```python
from build123d import *

# Parameters (mm, degrees)
SKETCH_1_R                = 44
EXTRUDE_1_DEPTH           = 80
CUT_EXTRUDE_START         = 5
SKETCH_2_W                = 23
SKETCH_2_H                = 72
CUT_EXTRUDE_5_DEPTH       = 97.350875675
SKETCH_3_W                = 20.9
SKETCH_3_H                = 40.9
CUT_EXTRUDE_6_DEPTH       = 120.436175424
EXTRUDE_2_DEPTH           = 75
SKETCH_7_R                = 6.5
CUT_EXTRUDE_7_DEPTH       = 4
CUT_EXTRUDE_START_2       = -4
SKETCH_8_R                = 6.5
CUT_EXTRUDE_8_DEPTH       = 4
CUT_EXTRUDE_9_REACH       = 105.057
SKETCH_9_R                = 5.5
CUT_EXTRUDE_10_DEPTH      = 120.436175424
CUT_EXTRUDE_10_DEPTH_BACK = 120.436175424
CUT_EXTRUDE_START_3       = -12
CUT_EXTRUDE_13_DEPTH      = 12
CUT_EXTRUDE_14_REACH      = 96.265
CUT_REVOLVE_1_ANGLE       = 180
CUT_REVOLVE_2_ANGLE       = 180
CUT_EXTRUDE_20_REACH      = 93.901


with BuildPart() as part:
    # 草图1 → 凸台-拉伸1 (new body)
    with BuildSketch(Plane(origin=(0, 0, 0), x_dir=(1, 0, 0), z_dir=(0, 1, 0))):
        with Locations(Location((0, 0, 0), (0, 0, 270))):
            Circle(SKETCH_1_R)
    extrude(amount=EXTRUDE_1_DEPTH)

    # 草图2 → 切除-拉伸5 (cut, through all)
    with BuildSketch(Plane(origin=(0, 0, 0), x_dir=(1, 0, 0), z_dir=(0, 1, 0)).offset(CUT_EXTRUDE_START)):
        with BuildLine():
            Line((33, 29.103264422), (33, -19.45))
            Line((33, -19.45), (39.467676648, -19.45))
            ThreePointArc((39.467676648, -19.45), (43.614744195, 5.809826917), (33, 29.103264422))
        make_face()
        with Locations((11.5, 8)):
            Rectangle(SKETCH_2_W, SKETCH_2_H)
    cut_extrude_5 = extrude(amount=CUT_EXTRUDE_5_DEPTH, mode=Mode.SUBTRACT)

    # 镜向1: 切除-拉伸5 across plane
    add(cut_extrude_5.mirror(Plane(origin=(0, 0, 0), x_dir=(0, 0, 1), z_dir=(1, 0, 0))), mode=Mode.SUBTRACT)

    # 草图3 → 切除-拉伸6 (cut, through all)
    with BuildSketch(Plane(origin=(33, 0, 0), x_dir=(0, 0, -1), z_dir=(1, 0, 0))):
        with Locations((-7, 33)):
            Rectangle(SKETCH_3_W, SKETCH_3_H)
    extrude(amount=-CUT_EXTRUDE_6_DEPTH, mode=Mode.SUBTRACT)

    # 草图6 → 凸台-拉伸2 (add)
    with BuildSketch(Plane(origin=(0, 5, 0), x_dir=(1, 0, 0), z_dir=(0, 1, 0))):
        with BuildLine():
            Line((-8.2, 43.229156827), (-8.2, -28))
            Line((-8.2, -28), (3.8, -28))
            Line((3.8, -28), (3.8, 43.835601969))
            ThreePointArc((3.8, 43.835601969), (-2.220798038, 43.943919444), (-8.2, 43.229156827))
        make_face()
    extrude(amount=EXTRUDE_2_DEPTH)

    # 草图7 → 切除-拉伸7 (cut)
    with BuildSketch(Plane(origin=(3.8, 0, 0), x_dir=(0, 0, -1), z_dir=(1, 0, 0))):
        with Locations((-7, 43)):
            Circle(SKETCH_7_R)
    extrude(amount=-CUT_EXTRUDE_7_DEPTH, mode=Mode.SUBTRACT)

    # 草图8 → 切除-拉伸8 (cut)
    with BuildSketch(Plane.ZY.offset(8.2).offset(CUT_EXTRUDE_START_2)):
        with Locations(Location((7, 43, 0), (0, 0, 180))):
            Circle(SKETCH_8_R)
    extrude(amount=CUT_EXTRUDE_8_DEPTH, mode=Mode.SUBTRACT)

    # 草图9 → 切除-拉伸9 (cut, up to next)
    with BuildSketch(Plane(origin=(3.8, 0, 0), x_dir=(0, 0, -1), z_dir=(1, 0, 0)), mode=Mode.PRIVATE) as cut_extrude_9_sk1:
        with Locations((-7, 43)):
            Circle(SKETCH_9_R)
    cut_extrude_9_tool1 = extrude(cut_extrude_9_sk1.sketch, amount=-CUT_EXTRUDE_9_REACH, mode=Mode.PRIVATE) & part.part
    add(cut_extrude_9_tool1.solids().sort_by_distance((3.8, 43, 7))[0], mode=Mode.SUBTRACT)

    # 草图10 → 切除-拉伸10 (cut, two sides: drawn at the far end of the back side and taken through both)
    with BuildSketch(Plane(origin=(33, 0, 0), x_dir=(0, 0, -1), z_dir=(1, 0, 0)).offset(-CUT_EXTRUDE_10_DEPTH_BACK)):
        with BuildLine():
            Line((44, 80), (44, 65))
            Line((44, 65), (-7, 65))
            ThreePointArc((-7, 65), (-19.069252989, 61.393834083), (-27.181803363, 51.757557481))
            Line((-27.181803363, 51.757557481), (-44, 13))
            Line((-44, 13), (-44, 80))
            Line((-44, 80), (44, 80))
        make_face()
    extrude(amount=CUT_EXTRUDE_10_DEPTH + CUT_EXTRUDE_10_DEPTH_BACK, mode=Mode.SUBTRACT)

    # 草图18 → 切除-拉伸13 (cut)
    with BuildSketch(Plane.ZY.offset(8.2).offset(CUT_EXTRUDE_START_3)):
        with BuildLine():
            ThreePointArc((-16.994306564, 43.522735592), (-16.113193955, 49.463765557), (-13.784609691, 55))
            ThreePointArc((-13.784609691, 55), (-8.989980812, 60.897500207), (-2.591663047, 65))
            Line((-2.591663047, 65), (-21.495613698, 65))
            ThreePointArc((-21.495613698, 65), (-26.943692062, 54.992738185), (-28.991459846, 43.784103388))
            Line((-28.991459846, 43.784103388), (-16.994306564, 43.522735592))
        make_face()
    extrude(amount=CUT_EXTRUDE_13_DEPTH, mode=Mode.SUBTRACT)

    # 草图19 → 切除-拉伸14 (cut, up to next)
    with BuildSketch(Plane.ZY.offset(8.2), mode=Mode.PRIVATE) as cut_extrude_14_sk1:
        with BuildLine():
            Line((-25.784609691, 34.215390309), (-20.368569743, 43.596246675))
            Line((-20.368569743, 43.596246675), (-28.991459846, 43.784103388))
            ThreePointArc((-28.991459846, 43.784103388), (-26.943692062, 54.992738185), (-21.495613698, 65))
            Line((-21.495613698, 65), (-43.229156827, 65))
            Line((-43.229156827, 65), (-43.229156827, 44.287004294))
            Line((-43.229156827, 44.287004294), (-25.784609691, 34.215390309))
        make_face()
    cut_extrude_14_tool1 = extrude(cut_extrude_14_sk1.sketch, amount=-CUT_EXTRUDE_14_REACH, mode=Mode.PRIVATE) & part.part
    # 草图19 → 切除-拉伸14 (cut, up to next)
    with BuildSketch(Plane.ZY.offset(8.2), mode=Mode.PRIVATE) as cut_extrude_14_sk2:
        with BuildLine():
            Line((-20.368569743, 43.596246675), (-13.784609691, 55))
            Line((-13.784609691, 55), (-13.784609691, 93.841822502))
            Line((-13.784609691, 93.841822502), (-75.156898342, 93.841822502))
            Line((-75.156898342, 93.841822502), (-75.156898342, 62.720494453))
            Line((-75.156898342, 62.720494453), (-43.229156827, 44.287004294))
            Line((-43.229156827, 44.287004294), (-43.229156827, 65))
            Line((-43.229156827, 65), (-21.495613698, 65))
            ThreePointArc((-21.495613698, 65), (-26.943692062, 54.992738185), (-28.991459846, 43.784103388))
            Line((-28.991459846, 43.784103388), (-20.368569743, 43.596246675))
        make_face()
    cut_extrude_14_tool2 = extrude(cut_extrude_14_sk2.sketch, amount=-CUT_EXTRUDE_14_REACH, mode=Mode.PRIVATE) & part.part
    add(cut_extrude_14_tool1.solids().sort_by_distance((-8.2, 51.836761, -33.537679))[0], mode=Mode.SUBTRACT)
    add(cut_extrude_14_tool2.solids().sort_by_distance((-8.2, 73.617285, -43.768646))[0], mode=Mode.SUBTRACT)

    # 草图24 → 切除-旋转1 (revolve, symmetric, cut)
    with BuildSketch(Plane(origin=(0, 43, 0), x_dir=(-1, 0, 0), z_dir=(0, -1, 0))) as cut_revolve_1_sk:
        Polygon((15.5, -31.8), (15.5, -34.8), (-15.5, -34.8), (-15.5, -31.8), (-15.5, -7), (-3.8, -7), (-3.8, -31.8), (8.2, -31.8), (8.2, -7), (15.5, -7), align=None)
    revolve(axis=Axis((-101.499852898, 43, 7), (1, 0, 0)), revolution_arc=CUT_REVOLVE_1_ANGLE / 2, mode=Mode.SUBTRACT)
    revolve(cut_revolve_1_sk.sketch, axis=Axis((-101.499852898, 43, 7), (-1, 0, 0)), revolution_arc=CUT_REVOLVE_1_ANGLE / 2, mode=Mode.SUBTRACT)

    # 草图26 → 切除-旋转2 (revolve, symmetric, cut)
    with BuildSketch(Plane(origin=(0, 43, 0), x_dir=(1, 0, 0), z_dir=(0, 1, 0))) as cut_revolve_2_sk:
        Polygon((-15.5, -34.551556537), (-23, -29.3), (-23, -28), (-15.5, -28), align=None)
        Polygon((15.5, -34.551556537), (23, -29.3), (23, -28), (15.5, -28), align=None)
    revolve(axis=Axis((-28, 43, 7), (1, 0, 0)), revolution_arc=CUT_REVOLVE_2_ANGLE / 2, mode=Mode.SUBTRACT)
    revolve(cut_revolve_2_sk.sketch, axis=Axis((-28, 43, 7), (-1, 0, 0)), revolution_arc=CUT_REVOLVE_2_ANGLE / 2, mode=Mode.SUBTRACT)

    # 草图28 → 切除-拉伸20 (cut, up to next)
    with BuildSketch(Plane(origin=(3.8, 0, 0), x_dir=(0, 0, -1), z_dir=(1, 0, 0)), mode=Mode.PRIVATE) as cut_extrude_20_sk1:
        with BuildLine():
            ThreePointArc((-7, 15.2), (-6.737382717, 15.201240456), (-6.474788871, 15.204961715))
            Line((-6.474788871, 15.204961715), (-5.365047446, 18.253951222))
            ThreePointArc((-5.365047446, 18.253951222), (-6.182078765, 18.213491475), (-7, 18.2))
            Line((-7, 18.2), (-7, 15.2))
        make_face()
    cut_extrude_20_tool1 = extrude(cut_extrude_20_sk1.sketch, amount=-CUT_EXTRUDE_20_REACH, mode=Mode.PRIVATE) & part.part
    add(cut_extrude_20_tool1.solids().sort_by_distance((3.8, 16.966985, 6.413126))[0], mode=Mode.SUBTRACT)


solid = part.part
```
Check sheet for the modelled part. Datum: model origin and axes. Units: mm. A direction names the side the tool comes from. Coordinates: 2 decimals unless noted, no trailing zeros. Order: outer loops, then holes, each group sorted by start corner. A loop starts at its lowest first (then second) coordinate and runs counter-clockwise, first axis right, second up. Notation, with made-up numbers: (45.25, -35.75) -> (77.25, -35.75) arc R30 cw to (77.25, -6.75) -> close; hole circle Ø8 at (16, 29). An arc over 180 degrees is marked (long way). Write each question's results on one line, items separated by ' | '. Start each with the question number.
1) Section check B-B (x = -27.5). Enter the section's corners in (y, z).
2) Section check D-D (z = -32.5). Enter the section's corners in (x, y).
3) Section check A-A (y = 21). Enter the section's corners in (x, z).
4) Draft check along Z on faces 1 (the face through (-2.28, 46.58, 29.43)), 2 (the face through (-2.284, 38.84, -23.115)), 3 (the face through (23, 35, -4)). Enter one of: pulls with the +Z half, pulls with the -Z half, needs draft (parallel to the pull), parting line crosses it, or undercut.
5) Depth check by flat-ended pin: pin 1 (10 mm diameter, centred on x = -26, y = 10, fed in from -Z); pin 2 (15.5 mm diameter, centred on x = 11, y = 18.5, fed in from -Z); pin 3 (4 mm diameter, centred on y = 43.5, z = -22.5, fed in from -X). Enter the tip coordinate at first touch or a pass-through.
6) Material ranges on line 1 along X through (y, z) = (10.5, -4); line 2 along X through (y, z) = (7.5, 19.5); line 3 along Z through (x, y) = (-6.8, 43), recorded low to high.
7) Set-up check for faces 4 (the face through (37, 5, -5)), 5 (the face through (-15, 5, -8)), 6 (the face through (-28, 53.45, 7)): record each of +Z, -Z, +X, -X, +Y, -Y from which the full face is reachable in a straight line by a thin tool's end or side.
8) Section check C-C (z = 22.5). Enter the section's corners in (x, y), and give its area (3 significant figures).
Checked values:
1) outline: (0, -34.35) -> (65, -34.35) -> (65, 7) arc R22 ccw to (51.76, 27.18) -> (35.24, 34.35) -> (0, 34.35) -> close; hole (12.55, -3.45) -> (53.45, -3.45) -> (53.45, 17.45) -> (12.55, 17.45) -> close
2) outline: (-29.66, 0) -> (29.66, 0) -> (29.66, 65) -> (23, 65) -> (23, 5) -> (3.8, 5) -> (3.8, 38.09) -> (-8.2, 38.09) -> (-8.2, 5) -> (-23, 5) -> (-23, 65) -> (-29.66, 65) -> close
3) outline: (-39.47, 19.45) -> (-33, 19.45) -> (-33, 17.45) -> (-23, 17.45) -> (-23, 28) -> (-8.2, 28) -> (-8.2, 24) -> (3.8, 24) -> (3.8, 28) -> (23, 28) -> (23, 17.45) -> (33, 17.45) -> (33, 19.45) -> (39.47, 19.45) arc R44 ccw to (17.13, 40.53) -> (-17.13, 40.53) arc R44 ccw to start; (-33, -29.1) arc R44 ccw to (-23, -37.51) -> (-23, -3.45) -> (-33, -3.45) -> close; (-8.2, -43.23) arc R44 ccw to (3.8, -43.84) -> (3.8, 18.45) -> (-8.2, 18.45) -> close; (23, -37.51) arc R44 ccw to (33, -29.1) -> (33, -3.45) -> (23, -3.45) -> close
4) face 1: pulls with the +Z half | face 2: undercut | face 3: needs draft
5) pin 1: z = -37.51 | pin 2: z = -43.88 | pin 3: x = -33
6) line 1: -33 to -23, -8.2 to 3.8, 23 to 33 | line 2: -39.44 to -23, -8.2 to 3.8, 23 to 39.44 | line 3: -43.47 to -41, -20.71 to 0.5, 13.5 to 30.98
7) face 4: -Z, +X, +Y | face 5: -Z, +Y | face 6: -X
8) outline: (-37.81, 0) -> (37.81, 0) -> (37.81, 58.61) -> (23, 58.61) -> (23, 5) -> (3.8, 5) -> (3.8, 19.92) -> (-8.2, 19.92) -> (-8.2, 5) -> (-23, 5) -> (-23, 58.61) -> (-37.81, 58.61) -> close; (-8.2, 23.64) -> (3.8, 23.64) -> (3.8, 58.61) -> (-8.2, 58.61) -> close | area: 2,570 mm²
